The listing builds one solid part. Answer for the finished solid, in the listing's coordinates (mm). Round coordinates to 2 decimals unless told otherwise and drop trailing zeros. Write each loop counter-clockwise with the first axis right and the second up, starting at its lowest first coordinate (ties: lowest second). Pieces come first, ordered by that corner, then holes. Notation, with made-up numbers: (61, 2.25) - (104, 2.25) arc R23 cw to (104, 18.25) - close; hole circle Ø6 at (27, 83). An arc over 180 degrees is marked (long way). Return JSON: item names as keys, results as strings. Group by question number.
(1) This flat-tipped pin is pushed along its axis until it touches: pin 1 (4 mm diameter, centred on x = 90.84, y = 60.73, fed in from +Z). Where does it stop, or does it pass through?
(2) Section A-A, the plane y = 26 is taken. Write down the section's boundary in (x, z).
(3) Section B-B, the plane x = 6 is taken. Write down the section's boundary in (y, z), then the cut area to 3 significant figures.
(4) Find the intervals of material crossed by line 1 along X through (y, z) = (26, 0.55); line 2 along Y through (x, z) = (6, 1.55); line 3 along X through (y, z) = (28, 1.2), in increasing order. Write a range as [from, to].
(5) Section D-D, the plane z = 0.25 is taken. Write down the section's boundary in (x, y).
(6) Determine the mould class of faces 1 (the flat face through (77, 26, 0)), 2 (the flat face through (124.76, 48.08, 0.79)), 3 (the cylindrical face through (6.74, 34.58, 0.74)), 4 (the cylindrical face through (50.366, 61.214, 0.74)) for opening direction Y: +Y half, -Y half, draft (parallel to the pull), parting line (faces both ways), or undercut.
(7) Section C-C, the plane y = 6 is taken. Write down the section's boundary in (x, z), then the cut area to 3 significant figures.
```python
from build123d import *

# Parameters (mm, degrees)
SKETCH1_R           = 1.6
BOSS_EXTRUDE1_DEPTH = 1.6
FILLET1_R           = 3
SKETCH2_R           = 3
CUT_EXTRUDE1_DEPTH  = 0.1


with BuildPart() as part:
    # Sketch1 → Boss-Extrude1 (new body)
    with BuildSketch(Plane.XY):
        Polygon((0, 0), (157, 0), (157, 29.464101615), (92.447441117, 66.733538863), (47.232050808, 66.733538863), (0, 39.464101615), align=None)
        with Locations((6, 36)):
            Circle(SKETCH1_R, mode=Mode.SUBTRACT)
        with Locations((6, 6)):
            Circle(SKETCH1_R, mode=Mode.SUBTRACT)
        with Locations((151, 6)):
            Circle(SKETCH1_R, mode=Mode.SUBTRACT)
        with Locations((151, 26)):
            Circle(SKETCH1_R, mode=Mode.SUBTRACT)
        with Locations((90.839745962, 60.733538863)):
            Circle(SKETCH1_R, mode=Mode.SUBTRACT)
        with Locations((48.839745962, 60.733538863)):
            Circle(SKETCH1_R, mode=Mode.SUBTRACT)
    extrude(amount=BOSS_EXTRUDE1_DEPTH)

    # Fillet1
    fillet1_edges = [part.edges().sort_by_distance(p)[0] for p in [
        (0, 39.464101615, 0.8),
        (47.232050808, 66.733538863, 0.8),
        (92.447441117, 66.733538863, 0.8),
        (157, 29.464101615, 0.8),
        (157, 0, 0.8),
        (0, 0, 0.8),
    ]]
    fillet(fillet1_edges, radius=FILLET1_R)

    # Sketch2 → Cut-Extrude1 (cut)
    with BuildSketch(Plane.XY.offset(1.6)):
        with Locations((6, 6)):
            Circle(SKETCH2_R)
        with Locations((6, 36)):
            Circle(SKETCH2_R)
        with Locations((48.839745962, 60.733538863)):
            Circle(SKETCH2_R)
        with Locations((90.839745962, 60.733538863)):
            Circle(SKETCH2_R)
        with Locations((151, 26)):
            Circle(SKETCH2_R)
        with Locations((151, 6)):
            Circle(SKETCH2_R)
    extrude(amount=-CUT_EXTRUDE1_DEPTH, mode=Mode.SUBTRACT)


solid = part.part
```
Working result:
{
 "1": {"pin 1": "stops at z = 1.5"},
 "2": {"outline": "(0, 0) - (149.4, 0) - (149.4, 1.5) - (148, 1.5) - (148, 1.6) - (0, 1.6) - close; (152.6, 0) - (157, 0) - (157, 1.6) - (154, 1.6) - (154, 1.5) - (152.6, 1.5) - close"},
 "3": {"outline": "(0, 0) - (4.4, 0) - (4.4, 1.5) - (3, 1.5) - (3, 1.6) - (0, 1.6) - close; (7.6, 0) - (34.4, 0) - (34.4, 1.5) - (33, 1.5) - (33, 1.6) - (9, 1.6) - (9, 1.5) - (7.6, 1.5) - close; (37.6, 0) - (42.93, 0) - (42.93, 1.6) - (39, 1.6) - (39, 1.5) - (37.6, 1.5) - close", "area": "57.9 mm^2"},
 "4": {"line 1": "x = [0, 149.4], [152.6, 157]", "line 2": "y = [0, 3], [9, 33], [39, 42.93]", "line 3": "x = [0, 156.99]"},
 "5": {"outline": "(0, 3) arc R3 ccw to (3, 0) - (154, 0) arc R3 ccw to (157, 3) - (157, 27.73) arc R3 ccw to (155.5, 30.33) - (93.14, 66.33) arc R3 ccw to (91.64, 66.73) - (48.04, 66.73) arc R3 ccw to (46.54, 66.33) - (1.5, 40.33) arc R3 ccw to (0, 37.73) - close; hole circle Ø3.2 at (6, 6); hole circle Ø3.2 at (6, 36); hole circle Ø3.2 at (48.84, 60.73); hole circle Ø3.2 at (90.84, 60.73); hole circle Ø3.2 at (151, 6); hole circle Ø3.2 at (151, 26)"},
 "6": {"face 1": "draft", "face 2": "+Y half", "face 3": "undercut", "face 4": "undercut"},
 "7": {"outline": "(0, 0) - (4.4, 0) - (4.4, 1.5) - (3, 1.5) - (3, 1.6) - (0, 1.6) - close; (7.6, 0) - (149.4, 0) - (149.4, 1.5) - (148, 1.5) - (148, 1.6) - (9, 1.6) - (9, 1.5) - (7.6, 1.5) - close; (152.6, 0) - (157, 0) - (157, 1.6) - (154, 1.6) - (154, 1.5) - (152.6, 1.5) - close", "area": "240 mm^2"}
}
